Geometry check sheet. Reference: the model listing, model coordinates, mm. Face numbers are marked on the shaded views. Give positions to 0.01 mm unless a question says otherwise; leave off trailing zeros. Order: outer loops, then holes, each group sorted by start corner. A loop starts at its lowest first (then second) coordinate and runs counter-clockwise, first axis right, second up. Notation, with made-up numbers: M 65.25,-4 L 98.25,-4 A17 cw 98.25,19 Z; hole C -34.5,23 d4. An arc over 180 degrees is marked long. Answer as CSV lines item,"result". Start each with the question number.
Q1. Mould release check, pull along Z, two halves, no side actions. Record for the marked faces 1, 2 and 3: +Z half, -Z half, draft (parallel to the pull), parting line (faces both ways), or undercut.
Q2. Thickness scan on line 1 (Z direction, x = 0, y = -17); line 2 (Z direction, x = 65, y = -9); line 3 (X direction, y = -33, z = -1.5). Record the ranges inside material, lowest first.
Q3. Go/stop test with flat-tipped pins: pin 1 (12 mm diameter, centred on y = -42, z = 18, fed in from -X); pin 2 (12 mm diameter, centred on y = -23.5, z = 0, fed in from -X); pin 3 (12 mm diameter, centred on x = 8.5, y = -20.5, fed in from +Z). Record where each tip stops, or that it passes through.
Q4. Section check B-B, the plane z = -8.5. Count the separate pieces of the cut face and the enclosed holes in it, then the cut area to 3 significant figures.
Q5. Section check A-A, the plane y = -4. Record the boundary of the cut face in (x, z).
```python
from build123d import *

# Parameters (mm, degrees)
F0_R     = 15
F0_R_2   = 10
F1_DEPTH = 25
F2_DEPTH = 50
F3_SIZE  = 3
F4_R     = 2


with BuildPart() as f1:
    # F0 (on Front) → F1 (new body)
    with BuildSketch(Plane.XZ):
        with BuildLine():
            ThreePointArc((6.0280672627, -29.3881337461), (23.2469569824, -18.9625681557), (30, 0))
            ThreePointArc((30, 0), (23.2980522028, 18.899755648), (6.186615763, 29.3551662472))
            ThreePointArc((6.186615763, 29.3551662472), (-29.9998907311, 0.0809698754), (6.0280672627, -29.3881337461))
        make_face()
        Circle(F0_R, mode=Mode.SUBTRACT)
        with BuildLine():
            ThreePointArc((6.186615763, 29.3551662472), (23.2980522028, 18.899755648), (30, 0))
            ThreePointArc((30, 0), (23.2469569824, -18.9625681557), (6.0280672627, -29.3881337461))
            Line((6.0280672627, -29.3881337461), (64.0985580176, -17.476767503))
            ThreePointArc((64.0985580176, -17.476767503), (47.5088589909, -0.5567640428), (62.9888960495, 17.384057665))
            Line((62.9888960495, 17.384057665), (6.186615763, 29.3551662472))
        make_face()
        with BuildLine():
            ThreePointArc((82.5, 0), (76.6416425144, 13.0660690174), (62.9888960495, 17.384057665))
            ThreePointArc((62.9888960495, 17.384057665), (47.5088589909, -0.5567640428), (64.0985580176, -17.476767503))
            ThreePointArc((64.0985580176, -17.476767503), (77.0514473261, -12.6890747238), (82.5, 0))
        make_face()
        with Locations((65, 0)):
            Circle(F0_R_2, mode=Mode.SUBTRACT)
    extrude(amount=F1_DEPTH)

    # F0 (on Front) → F2 (join)
    with BuildSketch(Plane.XZ):
        with BuildLine():
            ThreePointArc((6.0280672627, -29.3881337461), (23.2469569824, -18.9625681557), (30, 0))
            ThreePointArc((30, 0), (23.2980522028, 18.899755648), (6.186615763, 29.3551662472))
            ThreePointArc((6.186615763, 29.3551662472), (-29.9998907311, 0.0809698754), (6.0280672627, -29.3881337461))
        make_face()
        Circle(F0_R, mode=Mode.SUBTRACT)
    extrude(amount=F2_DEPTH)

    # F3
    f3_edges = [f1.edges().sort_by_distance(p)[0] for p in [
        (-15, -50, 0),
        (55, -25, 0),
    ]]
    chamfer(f3_edges, length=F3_SIZE)

    # F4
    f4_edges = [f1.edges().sort_by_distance(p)[0] for p in [
        (-6.028067, -50, 29.388134),
        (35.063313, 0, -23.432451),
    ]]
    fillet(f4_edges, radius=F4_R)


solid = f1.part
```
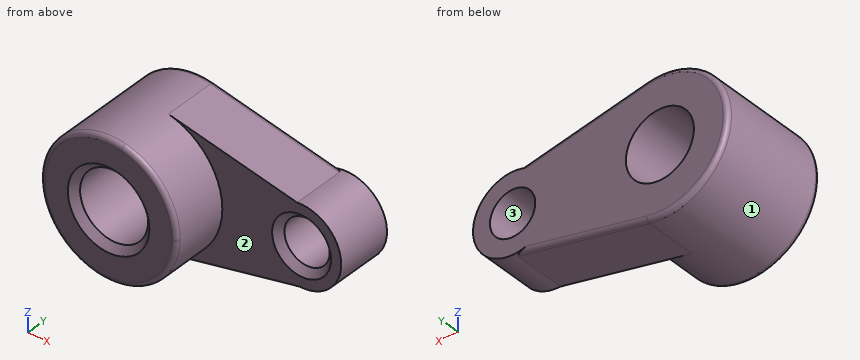
Answer block:
1,face 1,"parting line"
1,face 2,"draft"
1,face 3,"undercut"
2,line 1,"z = -30 to -15, 15 to 30"
2,line 2,"z = -17.5 to -10, 10 to 17.5"
2,line 3,"x = -29.96 to -14.92, 14.92 to 29.96"
3,pin 1,"stops at x = -27.5"
3,pin 2,"stops at x = -30"
3,pin 3,"stops at z = 29.9"
4,separate pieces,"3"
4,enclosed holes,"0"
4,area,"2,640 mm2"
5,outline,"M 6.03,-29.39 L 64.1,-17.48 A17.5 ccw long 62.99,17.38 L 6.19,29.36 A30 ccw long Z; hole C 0,0 d30; hole C 65,0 d20"
